Answer from the drawing. Dimensions are ordinates in mm from the lowest x, y and z of the part. A direction names the side the tool comes from. Coordinates: 2 decimals unless noted, no trailing zeros. Write each loop counter-clockwise with the first axis right and the second up, starting at its lowest first coordinate (ties: lowest second). Pieces come first, ordered by that corner, then holes.
(1) For a pull along Z with two mould halves and no side action, classify the marked faces 1, 2 and 3 as +Z half, -Z half, draft (parallel to the pull), parting line (faces both ways), or undercut.
(2) Which of the six approach directions +Z, -Z, +X, -X, +Y, -Y give full straight-line access (tool end or side, diameter ignored) to the marked faces 4 and 5?
(3) The part is cut by section B-B on z = 6. Determine the outline of the cut face in (x, y) (1 decimal).
(4) The part is cut by section A-A on x = 4.5. Determine the outline of the cut face in (y, z), plus the area to 3 significant figures.
(5) Straight lines are drawn through the part: line 1 (X direction, y = 0.7, z = 21) (1 decimal); line 2 (Z direction, x = 4.75, y = 0.4); line 3 (X direction, y = 1.05, z = 34) (1 decimal). For each, find the intervals that lie inside material, in ascending order.
(6) The part is cut by section C-C on y = 2.65. Determine the outline of the cut face in (x, z) (1 decimal).
(7) The part is cut by section D-D on z = 24. Determine the outline of the cut face in (x, y) (1 decimal).
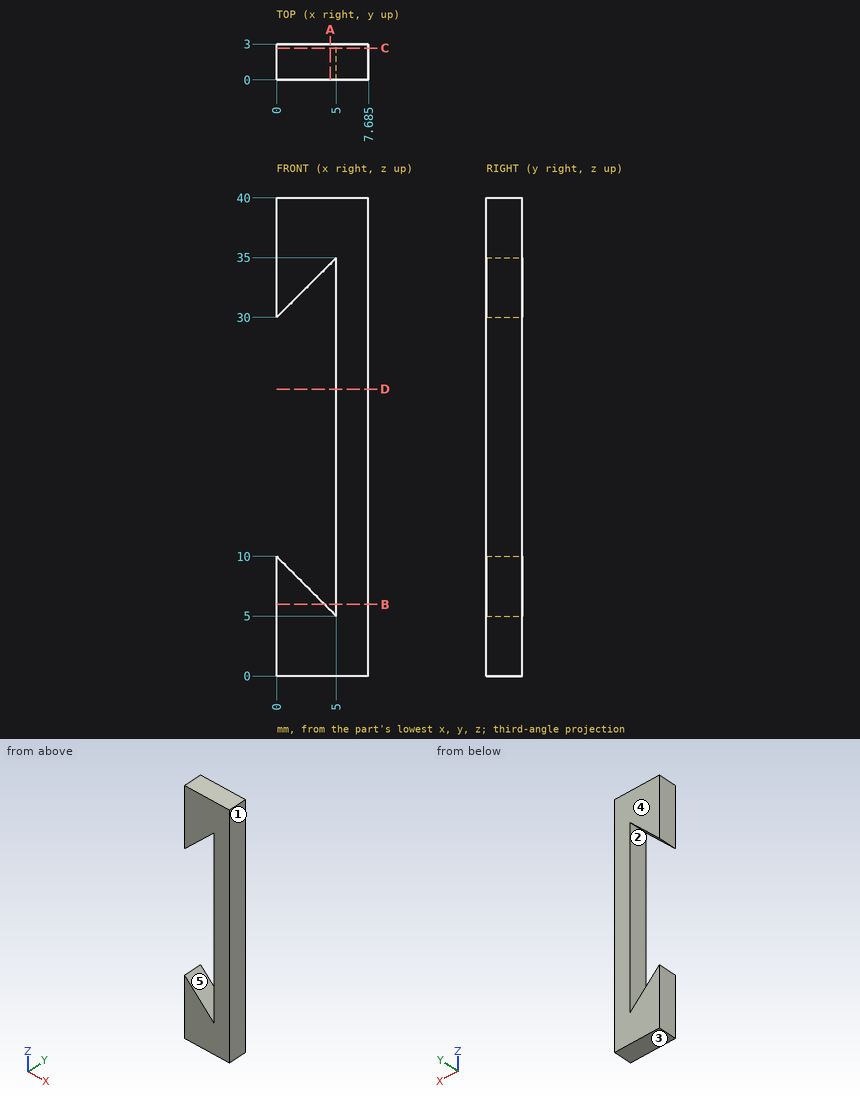
Model answer:
1. face 1: draft
1. face 2: undercut
1. face 3: -Z half
2. face 4: +Z, -Z, +X, -X, +Y
2. face 5: +Y, -Y
3. outline: (0, 0) - (4, 0) - (4, 3) - (0, 3) - close; (5, 0) - (7.7, 0) - (7.7, 3) - (5, 3) - close
4. outline: (0, 0) - (3, 0) - (3, 5.5) - (0, 5.5) - close; (0, 34.5) - (3, 34.5) - (3, 40) - (0, 40) - close
4. area: 33.0 mm2
5. line 1: x = 5 to 7.7
5. line 2: z = 0 to 5.25, 34.75 to 40
5. line 3: x = 0 to 4, 5 to 7.7
6. outline: (0, 0) - (7.7, 0) - (7.7, 40) - (0, 40) - (0, 30) - (5, 35) - (5, 5) - (0, 10) - close
7. outline: (5, 0) - (7.7, 0) - (7.7, 3) - (5, 3) - close
